Input: dimensioned drawing with shaded views. Units: mm. Origin: part minimum x, y, z. A direction names the side the tool comes from. Coordinates: 2 decimals unless noted, no trailing zeros. Order: outer loops, then holes, each group sorted by start corner. A loop starts at its lowest first (then second) coordinate and runs counter-clockwise, first axis right, second up. Notation, with made-up numbers: M 60,73 L 110,73 A30 cw 110,105 Z; hole C 6,14.5 d11. An arc over 180 degrees is marked long. Write item = value, one per line.
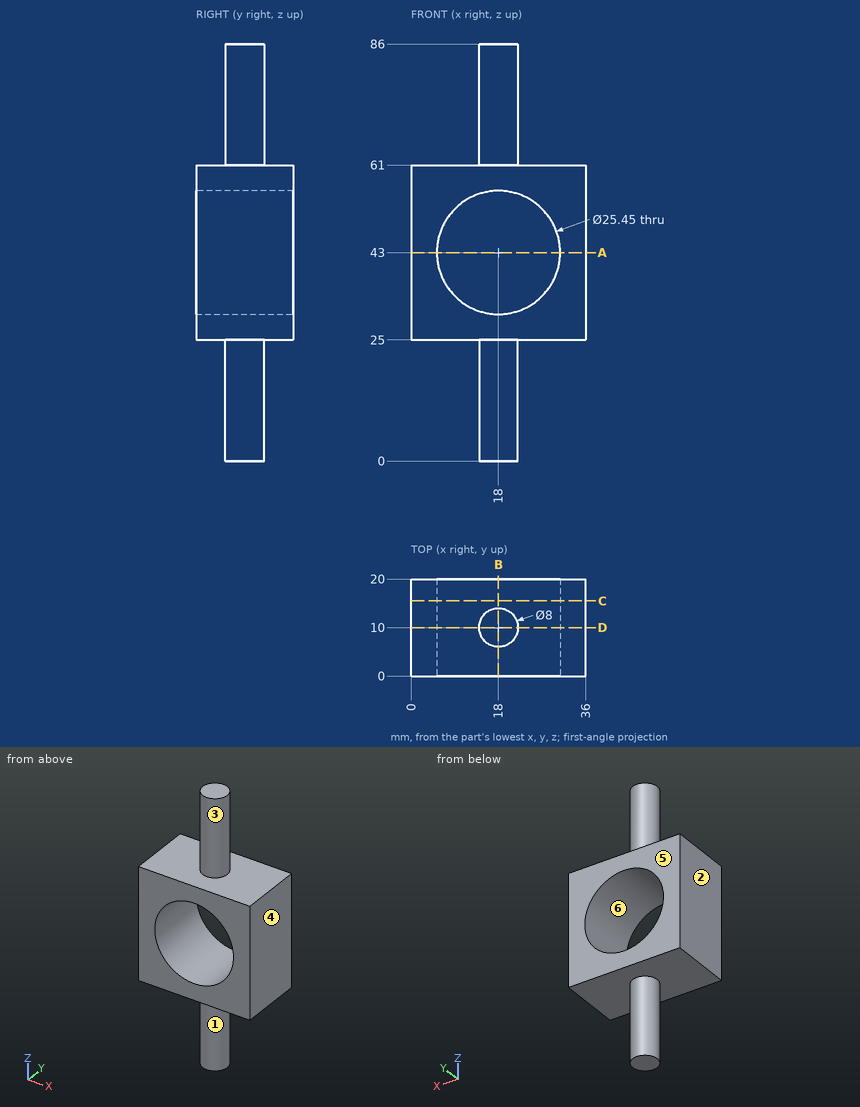
1) Line query: L1, parallel to X at y = 5.25, z = 43 (3 decimals); L2, parallel to Z at x = 2, y = 2.25; L3, parallel to Z at x = 11, y = 2. Output: solid intervals per line, ascending.
Numbers:
L1 = 0 to 5.275, 30.725 to 36
L2 = 25 to 61
L3 = 25 to 32.37, 53.63 to 61
2) Pin query (flat end, axial travel): pin 1 (10 mm diameter, centred on x = 29, y = 11, fed in from -Z); pin 2 (6 mm diameter, centred on y = 5.5, z = 77, fed in from -X); pin 3 (8 mm diameter, centred on x = 17.5, z = 74, fed in from +Y). Return the tip coordinate at first contact, or that it passes through.
Numbers:
pin_1 = 25
pin_2 = 14.29
pin_3 = 14
3) Set-up query: the marked faces 1, 2 and 3. Return all of +Z, -Z, +X, -X, +Y, -Y with unobstructed straight access to the full face (end or side cutting, diameter ignored); none if empty.
Numbers:
face_1 = -Z
face_2 = +Z, -Z, -X, +Y, -Y
face_3 = +Z
4) Section C-C, the plane y = 15.5. Return loops of the section in (x, z) (3 decimals), and give its area (3 significant figures).
Numbers:
outline = M 0,25 L 36,25 L 36,61 L 0,61 Z; hole C 18,43 d25.45
area = 787 mm²
5) Mould query, pull axis X, two halves, no side actions, for the marked faces 4, 5 and 6. Classes: pulls with the +X half, pulls with the -X half, needs draft (parallel to the pull), parting line crosses it, or undercut.
Numbers:
face_4 = pulls with the +X half
face_5 = needs draft
face_6 = undercut
6) Section D-D, the plane y = 10. Return loops of the section in (x, z) (3 decimals).
Numbers:
outline = M 0,25 L 14,25 L 14,0 L 22,0 L 22,25 L 36,25 L 36,61 L 22,61 L 22,86 L 14,86 L 14,61 L 0,61 Z; hole C 18,43 d25.45
7) Section A-A, the plane z = 43. Return loops of the section in (x, y) (3 decimals), and give its area (3 significant figures).
Numbers:
outline = M 0,0 L 5.275,0 L 5.275,20 L 0,20 Z; M 30.725,0 L 36,0 L 36,20 L 30.725,20 Z
area = 211 mm²
8) Section B-B, the plane x = 18. Return loops of the section in (y, z) (3 decimals), and give its area (3 significant figures).
Numbers:
outline = M 0,25 L 6,25 L 6,0 L 14,0 L 14,25 L 20,25 L 20,30.275 L 0,30.275 Z; M 0,55.725 L 20,55.725 L 20,61 L 14,61 L 14,86 L 6,86 L 6,61 L 0,61 Z
area = 611 mm²
